```python
from build123d import *

# Parameters (mm, degrees)
SKETCH2_W           = 38.1
SKETCH2_H           = 38.1
BOSS_EXTRUDE1_DEPTH = 1492.25
SHELL1_T            = -3.175
BOSS_EXTRUDE2_DEPTH = 6.35
SKETCH4_R           = 6.35
CUT_EXTRUDE1_DEPTH  = 1579.907420695
SKETCH7_R           = 1.5875


with BuildPart() as part:
    # Sketch2 → Boss-Extrude1 (new body)
    with BuildSketch(Plane(origin=(0, 0, 0), x_dir=(0, 0, -1), z_dir=(1, 0, 0))):
        Rectangle(SKETCH2_W, SKETCH2_H)
    extrude(amount=-BOSS_EXTRUDE1_DEPTH)

    # Shell1
    shell1_openings = [part.faces().sort_by_distance(p)[0] for p in [
        (-1492.25, 0, 0),
        (0, 0, 0),
    ]]
    offset(amount=SHELL1_T, openings=shell1_openings, kind=Kind.INTERSECTION)

    # Sketch3 → Boss-Extrude2 (add)
    with BuildSketch(Plane.XY.offset(19.05)):
        with BuildLine():
            Line((-1492.25, 19.05), (-1466.85, 19.05))
            Line((-1466.85, 19.05), (-1466.85, -19.05))
            Line((-1466.85, -19.05), (-1492.25, -19.05))
            Line((-1492.25, -19.05), (-1558.925, -19.05))
            ThreePointArc((-1558.925, -19.05), (-1577.975, 0), (-1558.925, 19.05))
            Line((-1558.925, 19.05), (-1492.25, 19.05))
        make_face()
    boss_extrude2 = extrude(amount=BOSS_EXTRUDE2_DEPTH)

    # Mirror1: Boss-Extrude2 across plane
    add(boss_extrude2.mirror(Plane.XY))

    # Sketch4 → Cut-Extrude1 (cut, through all)
    with BuildSketch(Plane.XY.offset(25.4)):
        with Locations((-1558.925, 0)):
            Circle(SKETCH4_R)
    extrude(amount=-CUT_EXTRUDE1_DEPTH, mode=Mode.SUBTRACT)

    # Sweep1: sweep along a path in Sketch5
    with BuildLine(Plane.XY) as sweep1_path:
        Line((-14.2875, -19.05), (-14.2875, -30.95625))
        ThreePointArc((-14.2875, -30.95625), (-7.14375, -38.1), (0, -30.95625))
    # Sketch7 → Sweep1 (sweep)
    with BuildSketch(Plane.XZ.offset(19.05)):
        with Locations((-14.2875, 0)):
            Circle(SKETCH7_R)
    sweep(path=sweep1_path.line)


solid = part.part
```
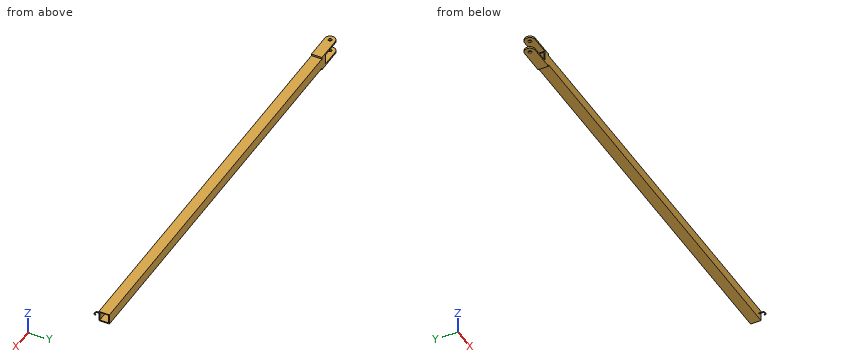
Verification items for the finished model (mm, model axes). Coordinates: 2 decimals unless noted, no trailing zeros. Loops run counter-clockwise (first coordinate to the right, second up) from the corner with the lowest first, then second, coordinate; pieces in that order, holes last. Notation, with made-up numbers: (31.5, 64) -> (65.5, 64) arc R23 cw to (65.5, 96) -> close; hole circle Ø4 at (49, 27.25). An arc over 180 degrees is marked (long way). Answer in a Markdown table with one row per item.
1) Section check A-A (x = -683.5). Record the cut outline in (y, z) (3 decimals), and give its area (3 significant figures).
The answers:
| item | result |
|---|---|
| outline | (-19.05, -19.05) -> (19.05, -19.05) -> (19.05, 19.05) -> (-19.05, 19.05) -> close; hole (-15.875, -15.875) -> (15.875, -15.875) -> (15.875, 15.875) -> (-15.875, 15.875) -> close |
| area | 444 mm2 |
2) Scan lines: line 1 along Z through (x, y) = (-795.5, -8) (3 decimals); line 2 along Y through (x, z) = (-437, 17.5). Record each from-to range of solid material in increasing order. Write a range as from..to.
The answers:
| item | result |
|---|---|
| line 1 | z = -19.05..-15.875, 15.875..19.05 |
| line 2 | y = -19.05..19.05 |
3) Depth check by flat-ended pin: P1, Ø7, axis at y = 3, z = -22.5, coming from the +X side; P2, Ø16, axis at x = -791.5, y = -3, coming from the +Z side; P3, Ø4, axis at y = -3, z = 15.5, coming from the -X side; P4, Ø11.5, axis at y = -5.5, z = -1, coming from the -X side. Enter the tip coordinate at first touch or a pass-through.
The answers:
| item | result |
|---|---|
| P1 | stops at x = 0 |
| P2 | stops at z = 19.05 |
| P3 | stops at x = -1492.25 |
| P4 | passes through |
